Work out the finished part from the listing and answer in its coordinate system (mm). A direction names the side the tool comes from. Give positions to 0.01 mm unless a question says otherwise; leave off trailing zeros. Loops run counter-clockwise (first coordinate to the right, second up) from the corner with the lowest first, then second, coordinate; pieces in that order, holes last. Notation, with made-up numbers: (60, -20.75) -> (73, -20.75) arc R11 ccw to (73, -13.75) -> close; hole circle Ø11 at (28.5, -15.5). An arc over 180 degrees is marked (long way). Answer as CSV lines item,"result". Start each with the question number.
1. Find section B-B, the plane x = 0. Give the vertices of the cut face in (y, z).
2. Find the intervals of material crossed by line 1 along Z through (x, y) = (-4, 52.5); line 2 along X through (y, z) = (17, 50); line 3 along Y through (x, z) = (15, 44), in increasing order.
3. A tool of negligible diameter and unlimited length cuts with its end or side. For faces 1 (the face through (0.1, 21, 68.2)), 2 (the face through (-7.57, 10.35, 34.4)), 3 (the face through (-0.252, 44.405, 59.332)), 4 (the face through (7.6, 10.35, 34.43)), 5 (the face through (0, 44, 61)), from which of +Z, -Z, +X, -X, +Y, -Y can it reach the whole face along a straight path? Write none if from no direction.
4. Find section D-D, the plane y = 17. Give the vertices of the cut face in (x, z).
5. Flat-ended cylindrical pins translate along their axes: pin 1 Ø1.3 at (x, z) = (-3, 62) entering from -Y; pin 2 Ø1.2 at (x, y) = (4, 15.5) entering from -Z; pin 3 Ø16.5 at (y, z) = (6, 29.5) entering from -X. Find the tip coordinate at first contact, or state that the pin passes through.
6. Find section A-A, the plane y = 52.5. Give the vertices of the cut face in (x, z).
7. Determine the mould class of faces 6 (the face through (9, 21, 37)), 7 (the face through (-0.252, 42.255, 12.861)), 8 (the face through (15.3, 25.6, 54.5)), 9 (the face through (-5, 10, 22)) for opening direction Y: +Y half, -Y half, draft (parallel to the pull), parting line (faces both ways), or undercut.
8. Find section C-C, the plane z = 39. Give the vertices of the cut face in (x, y).
from build123d import *

# Parameters (mm, degrees)
SKETCH017_AS_DRAWN_W                 = 6
SKETCH017_AS_DRAWN_H                 = 25
EXTRUDE002_DEPTH                     = 30
EXTRUDE002_ONTO_SKETCH017_ROLL_ANGLE = 90
SKETCH016_AS_DRAWN_R                 = 13.5
EXTRUDE001_DEPTH                     = 45
EXTRUDE001_ONTO_SKETCH016_ROLL_ANGLE = 90
EXTRUDE_DEPTH                        = 38
SKETCH014_W                          = 22
SKETCH014_H                          = 20
BOX_W                                = 36
BOX_H                                = 60
BOX_DEPTH                            = 70


with BuildPart() as arc_ext:
    # Sketch017 as drawn → Extrude002 (new)
    with BuildSketch(Plane.XY):
        with BuildLine():
            Line((9, 35), (20, 35))
            Line((20, 35), (20, 20))
            Line((20, 20), (7, 20))
            Line((7, 20), (7, 33))
            ThreePointArc((9, 35), (7.585786, 34.414214), (7, 33))
        make_face()
        with BuildLine():
            Line((-9, 35), (-20, 35))
            Line((-20, 35), (-20, 20))
            Line((-20, 20), (-7, 20))
            Line((-7, 20), (-7, 33))
            ThreePointArc((-7, 33), (-7.585786, 34.414214), (-9, 35))
        make_face()
        with Locations((0, 27.5)):
            Rectangle(SKETCH017_AS_DRAWN_W, SKETCH017_AS_DRAWN_H)
    extrude(amount=-EXTRUDE002_DEPTH)


with BuildPart() as arc_ext_1:
    # Extrude002 onto Sketch017 roll: moved
    add(arc_ext.part.rotate(Axis((0, 0, 0), (1, 0, 0)), EXTRUDE002_ONTO_SKETCH017_ROLL_ANGLE))


with BuildPart() as arc_ext_2:
    # Extrude002 onto Sketch017 placement: moved
    add(arc_ext_1.part)


with BuildPart() as arc_ext_3:
    # Extrude002 placement: moved
    add(arc_ext_2.part.moved(Location((0, -1, 0))))


with BuildPart() as fusion:
    # Sketch016 as drawn → Extrude001 (new)
    with BuildSketch(Plane.XY):
        with Locations((0, 50)):
            Circle(SKETCH016_AS_DRAWN_R)
    extrude(amount=-EXTRUDE001_DEPTH)


with BuildPart() as fusion_1:
    # Extrude001 onto Sketch016 roll: moved
    add(fusion.part.rotate(Axis((0, 0, 0), (1, 0, 0)), EXTRUDE001_ONTO_SKETCH016_ROLL_ANGLE))


with BuildPart() as fusion_2:
    # Extrude001 onto Sketch016 placement: moved
    add(fusion_1.part)


with BuildPart() as fusion_3:
    # Extrude001 placement: moved
    add(fusion_2.part.moved(Location((0, -1, 0))))

    # Fusion: union arc-ext
    add(arc_ext_3.part)


with BuildPart() as extrude_body:
    # Sketch → Extrude (new body)
    with BuildSketch(Plane.YZ):
        with BuildLine():
            Line((61, 60), (47.5, 60))
            ThreePointArc((47.5, 60), (42.196699, 57.803301), (40, 52.5))
            Line((40, 52.5), (40, 32.5))
            ThreePointArc((40, 32.5), (42.196699, 27.196699), (47.5, 25))
            Line((47.5, 25), (61, 25))
            Line((61, 25), (61, 60))
        make_face()
        with BuildLine():
            Line((61, 15), (47.5, 15))
            ThreePointArc((47.5, 15), (42.196699, 12.803301), (40, 7.5))
            Line((40, 7.5), (40, -2))
            Line((40, -2), (61, -2))
            Line((61, -2), (61, 15))
        make_face()
        with BuildLine():
            Line((30, 50), (30, -2))
            Line((30, -2), (-2, -2))
            Line((-2, -2), (-2, 22))
            Line((-2, 22), (21, 22))
            Line((21, 22), (21, 50))
            ThreePointArc((30, 50), (25.5, 54.5), (21, 50))
        make_face()
    extrude(amount=EXTRUDE_DEPTH)


with BuildPart() as extrude_body_1:
    # Extrude placement: moved
    add(extrude_body.part.moved(Location((-19, 0, 0))))


with BuildPart() as sweep_body:
    # Sweep: sweep along a path in Sketch015
    with BuildLine(Plane.XZ) as sweep_path:
        ThreePointArc((4, 40.834849), (0, 60), (-4, 40.834849))
    # Sketch014 → Sweep (sweep)
    with BuildSketch(Plane(origin=(0, -1, 0), x_dir=(0, 1, 0), z_dir=(1, 0, 0))):
        with Locations((11, 78)):
            Rectangle(SKETCH014_W, SKETCH014_H)
    sweep(path=sweep_path.line)


with BuildPart() as cut002:
    # Box → Box (new body)
    with BuildSketch(Plane(origin=(-18, 0, 0), x_dir=(1, 0, 0), z_dir=(0, 0, 1))):
        with Locations((18, 30)):
            Rectangle(BOX_W, BOX_H)
    extrude(amount=BOX_DEPTH)

    # Cut: cut Sweep body
    add(sweep_body.part, mode=Mode.SUBTRACT)

    # Cut001: cut Extrude body
    add(extrude_body_1.part, mode=Mode.SUBTRACT)

    # Cut002: cut Fusion
    add(fusion_3.part, mode=Mode.SUBTRACT)


solid = cut002.part
Resolved:
1,outline,"(0, 63.5) -> (44, 63.5) -> (44, 59.13) arc R7.5 cw to (47.5, 60) -> (60, 60) -> (60, 70) -> (21, 70) -> (21, 68) -> (0, 68) -> close; (30, 0) -> (40, 0) -> (40, 7.5) arc R7.5 cw to (47.5, 15) -> (60, 15) -> (60, 25) -> (47.5, 25) arc R7.5 cw to (40, 32.5) -> (40, 36.5) -> (30, 36.5) -> close"
2,line 1,"z = 15 to 25, 60 to 70"
2,line 2,"x = -18 to -13.5, 13.5 to 18"
2,line 3,"y = 0 to 21, 30 to 40"
3,face 1,"+Z, -Y"
3,face 2,"-Z, -X, -Y"
3,face 3,"+X, -X, +Y"
3,face 4,"-Z, +X, -Y"
3,face 5,"-Y"
4,outline,"(-9.95, 35) -> (-9, 35) arc R2 cw to (-7, 33) -> (-7, 22) -> (-3, 22) -> (-3, 36.84) arc R13.5 cw (long way) to (3, 36.84) -> (3, 22) -> (7, 22) -> (7, 33) arc R2 cw to (9, 35) -> (9.95, 35) arc R18 ccw (long way) to start"
5,pin 1,"stops at y = 44"
5,pin 2,"stops at z = 22"
5,pin 3,"stops at x = -13.19"
6,outline,"(-18, 15) -> (18, 15) -> (18, 25) -> (-18, 25) -> close; (-18, 60) -> (18, 60) -> (18, 70) -> (-18, 70) -> close"
7,face 6,"undercut"
7,face 7,"+Y half"
7,face 8,"undercut"
7,face 9,"draft"
8,outline,"(-18, 30) -> (-7.83, 30) -> (-7.83, 40) -> (-18, 40) -> close; (-14.25, 0) -> (-7.83, 0) -> (-7.83, 21) -> (-14.25, 21) -> close; (7.83, 0) -> (14.25, 0) -> (14.25, 21) -> (7.83, 21) -> close; (7.83, 30) -> (18, 30) -> (18, 40) -> (7.83, 40) -> close"
